from build123d import *

# Parameters (mm, degrees)
F0_W      = 232.5
F0_H      = 293
F1_DEPTH  = 200
F2_W      = 242.5
F2_H      = 5
F3_DEPTH  = 303
F5_DEPTH  = 25
F7_DEPTH  = 25
F9_DEPTH  = 210.001
F11_DEPTH = 210
F12_W     = 5
F12_H     = 82
F13_DEPTH = 232


with BuildPart() as f1:
    # F0 (on Front) → F1 (new body)
    with BuildSketch(Plane.XZ):
        Polygon((-92.2009944916, 239.5714490414), (-92.2009944916, 234.5714490414), (-92.2009944916, -63.4285509586), (150.2990055084, -63.4285509586), (150.2990055084, 239.5714490414), align=None)
        with Locations((29.0490055084, 88.0714490414)):
            Rectangle(F0_W, F0_H, mode=Mode.SUBTRACT)
    extrude(amount=F1_DEPTH)

    # F4 (on face) → F5 (cut)
    with BuildSketch(Plane.YZ.offset(150.2990055084)):
        with BuildLine():
            ThreePointArc((-42.5, 147.0714490414), (-44.6966991411, 152.3747499003), (-50, 154.5714490414))
            Line((-50, 154.5714490414), (-50, 147.0714490414))
            Line((-50, 147.0714490414), (-50, 139.5714490414))
            ThreePointArc((-50, 139.5714490414), (-44.6966991411, 141.7681481825), (-42.5, 147.0714490414))
        make_face()
        with BuildLine():
            ThreePointArc((-42.5, -24.9285509586), (-44.6966991411, -19.6252500997), (-50, -17.4285509586))
            Line((-50, -17.4285509586), (-50, -24.9285509586))
            Line((-50, -24.9285509586), (-50, -32.4285509586))
            ThreePointArc((-50, -32.4285509586), (-44.6966991411, -30.2318518175), (-42.5, -24.9285509586))
        make_face()
        with BuildLine():
            Line((-50, -24.9285509586), (-50, -17.4285509586))
            ThreePointArc((-50, -17.4285509586), (-57.5, -24.9285509586), (-50, -32.4285509586))
            Line((-50, -32.4285509586), (-50, -24.9285509586))
        make_face()
        with BuildLine():
            Line((-50, 147.0714490414), (-50, 154.5714490414))
            ThreePointArc((-50, 154.5714490414), (-57.5, 147.0714490414), (-50, 139.5714490414))
            Line((-50, 139.5714490414), (-50, 147.0714490414))
        make_face()
        with BuildLine():
            ThreePointArc((-142.5, 147.0714490414), (-144.6966991411, 152.3747499003), (-150, 154.5714490414))
            Line((-150, 154.5714490414), (-150, 147.0714490414))
            Line((-150, 147.0714490414), (-150, 139.5714490414))
            ThreePointArc((-150, 139.5714490414), (-144.6966991411, 141.7681481825), (-142.5, 147.0714490414))
        make_face()
        with BuildLine():
            ThreePointArc((-142.5, -24.9285509586), (-144.6966991411, -19.6252500997), (-150, -17.4285509586))
            Line((-150, -17.4285509586), (-150, -24.9285509586))
            Line((-150, -24.9285509586), (-150, -32.4285509586))
            ThreePointArc((-150, -32.4285509586), (-144.6966991411, -30.2318518175), (-142.5, -24.9285509586))
        make_face()
        with BuildLine():
            Line((-150, -24.9285509586), (-150, -17.4285509586))
            ThreePointArc((-150, -17.4285509586), (-157.5, -24.9285509586), (-150, -32.4285509586))
            Line((-150, -32.4285509586), (-150, -24.9285509586))
        make_face()
        with BuildLine():
            Line((-150, 147.0714490414), (-150, 154.5714490414))
            ThreePointArc((-150, 154.5714490414), (-157.5, 147.0714490414), (-150, 139.5714490414))
            Line((-150, 139.5714490414), (-150, 147.0714490414))
        make_face()
    extrude(amount=-F5_DEPTH, mode=Mode.SUBTRACT)

    # F6 (on face) → F7 (cut)
    with BuildSketch(Plane(origin=(0, 0, -63.4285509586), x_dir=(1, 0, 0), z_dir=(0, 0, -1))):
        with BuildLine():
            ThreePointArc((105.7990055084, 150), (113.2990055084, 142.5), (120.7990055084, 150))
            Line((120.7990055084, 150), (113.2990055084, 150))
            Line((113.2990055084, 150), (105.7990055084, 150))
        make_face()
        with BuildLine():
            Line((113.2990055084, 150), (120.7990055084, 150))
            ThreePointArc((120.7990055084, 150), (113.2990055084, 157.5), (105.7990055084, 150))
            Line((105.7990055084, 150), (113.2990055084, 150))
        make_face()
        with BuildLine():
            ThreePointArc((120.7990055084, 50), (113.2990055084, 57.5), (105.7990055084, 50))
            Line((105.7990055084, 50), (113.2990055084, 50))
            Line((113.2990055084, 50), (120.7990055084, 50))
        make_face()
        with BuildLine():
            Line((113.2990055084, 50), (105.7990055084, 50))
            ThreePointArc((105.7990055084, 50), (113.2990055084, 42.5), (120.7990055084, 50))
            Line((120.7990055084, 50), (113.2990055084, 50))
        make_face()
        with BuildLine():
            ThreePointArc((-19.2009944916, 50), (-21.3976936327, 55.3033008589), (-26.7009944916, 57.5))
            Line((-26.7009944916, 57.5), (-26.7009944916, 50))
            Line((-26.7009944916, 50), (-19.2009944916, 50))
        make_face()
        with BuildLine():
            Line((-26.7009944916, 50), (-26.7009944916, 57.5))
            ThreePointArc((-26.7009944916, 57.5), (-32.0042953505, 55.3033008589), (-34.2009944916, 50))
            Line((-34.2009944916, 50), (-26.7009944916, 50))
        make_face()
        with BuildLine():
            ThreePointArc((-26.7009944916, 142.5), (-21.3976936327, 144.6966991411), (-19.2009944916, 150))
            Line((-19.2009944916, 150), (-26.7009944916, 150))
            Line((-26.7009944916, 150), (-26.7009944916, 142.5))
        make_face()
        with BuildLine():
            Line((-26.7009944916, 150), (-19.2009944916, 150))
            ThreePointArc((-19.2009944916, 150), (-26.7009944916, 157.5), (-34.2009944916, 150))
            Line((-34.2009944916, 150), (-26.7009944916, 150))
        make_face()
        with BuildLine():
            Line((-26.7009944916, 142.5), (-26.7009944916, 150))
            Line((-26.7009944916, 150), (-34.2009944916, 150))
            ThreePointArc((-34.2009944916, 150), (-32.0042953505, 144.6966991411), (-26.7009944916, 142.5))
        make_face()
        with BuildLine():
            Line((-19.2009944916, 50), (-26.7009944916, 50))
            Line((-26.7009944916, 50), (-34.2009944916, 50))
            ThreePointArc((-34.2009944916, 50), (-26.7009944916, 42.5), (-19.2009944916, 50))
        make_face()
    extrude(amount=-F7_DEPTH, mode=Mode.SUBTRACT)



with BuildPart() as f3:
    # F2 (on face) → F3 (new body)
    with BuildSketch(Plane(origin=(0, 0, -63.4285509586), x_dir=(1, 0, 0), z_dir=(0, 0, -1))):
        with Locations((29.0490055084, 202.5)):
            Rectangle(F2_W, F2_H)
    extrude(amount=-F3_DEPTH)

    # F8 (on face) → F9 (cut, through all)
    with BuildSketch(Plane.XZ.offset(205)):
        with BuildLine():
            ThreePointArc((42.2990055084, 27.0714490414), (54.6733741792, 32.1970803706), (59.7990055084, 44.5714490414))
            ThreePointArc((59.7990055084, 44.5714490414), (29.9246368377, 56.9458177121), (42.2990055084, 27.0714490414))
        make_face()
    extrude(amount=-F9_DEPTH, mode=Mode.SUBTRACT)


with BuildPart() as f3b:
    # F2 (on face) → F3, piece 2 (new body)
    with BuildSketch(Plane(origin=(0, 0, -63.4285509586), x_dir=(1, 0, 0), z_dir=(0, 0, -1))):
        with Locations((29.0490055084, -2.5)):
            Rectangle(F2_W, F2_H)
    extrude(amount=-F3_DEPTH)


with BuildPart() as f1_1:
    add(f1.part)

    add(f3.part)  # F11 merges F3

    add(f3b.part)  # F11 merges F3b
    # F10 (on face) → F11 (join)
    with BuildSketch(Plane.XZ.offset(205)):
        Polygon((145.2990055084, -145.4285509586), (42.2990055084, -145.4285509586), (42.2990055084, -150.4285509586), (150.2990055084, -150.4285509586), (150.2990055084, -63.4285509586), (145.2990055084, -63.4285509586), align=None)
        Polygon((42.2990055084, -150.4285509586), (42.2990055084, -145.4285509586), (-87.2009944916, -145.4285509586), (-87.2009944916, -63.4285509586), (-92.2009944916, -63.4285509586), (-92.2009944916, -150.4285509586), align=None)
    extrude(amount=-F11_DEPTH)

    # F12 (on face) → F13 (join)
    with BuildSketch(Plane(origin=(145.2990055084, 0, 0), x_dir=(0, -1, 0), z_dir=(-1, 0, 0))):
        with Locations((-2.5, -104.4285509586)):
            Rectangle(F12_W, F12_H)
        with Locations((202.5, -104.4285509586)):
            Rectangle(F12_W, F12_H)
    extrude(amount=F13_DEPTH)


solid = f1_1.part
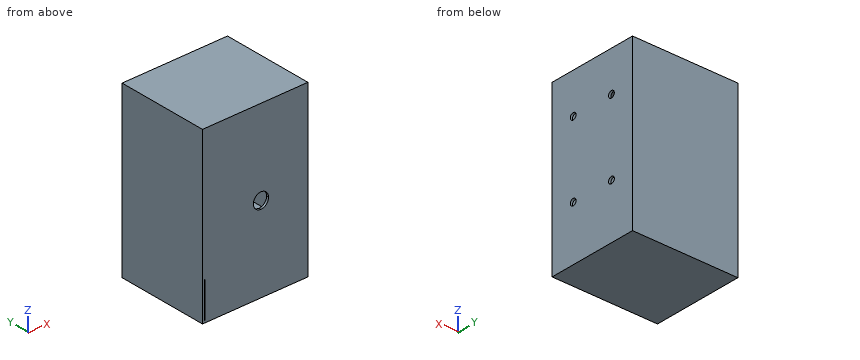
Could you check a few things on this model? Use its own coordinates, in mm. Give positions to 0.01 mm unless a question says otherwise; leave off trailing zeros. Write each loop counter-clockwise with the first axis right and the second up, starting at its lowest first coordinate (ties: lowest second). Pieces come first, ordered by that corner, then holes. Notation, with made-up numbers: (63.5, -20.5) -> (120.5, -20.5) arc R16 cw to (120.5, -10.5) -> close; hole circle Ø2 at (24, -2). An arc over 180 degrees is marked (long way). Answer as CSV lines item,"result". Start each with the question number.
(1) If we section it at C-C, the plane y = -92.5: Write out the boundary of the cut face in (x, z), and give its area (3 significant figures).
(2) I'm going to push a flat-ended pin straight in: pin 1 Ø12 at (y, z) = (-150, 147.07) entering from +X. Where does the tip first touch, or does it pass through?
(3) If we section it at D-D, the plane z = -116: Write out the boundary of the cut face in (x, y).
(4) If we section it at A-A, the plane z = 165: Write out the boundary of the cut face in (x, y), and give its area (4 significant figures).
(5) If we section it at B-B, the plane x = 130: Write out the boundary of the cut face in (y, z).
(6) Please list where these lines run through material, in increasing order: line 1 (Z direction, x = 124, y = -14); line 2 (Z direction, x = 149, y = -150); line 3 (Y direction, x = -1, z = 143.5).
Answer list:
1,outline,"(-92.2, -150.43) -> (150.3, -150.43) -> (150.3, 239.57) -> (-92.2, 239.57) -> close; hole (-87.2, -145.43) -> (145.3, -145.43) -> (145.3, -63.43) -> (-87.2, -63.43) -> close; hole (-87.2, -58.43) -> (145.3, -58.43) -> (145.3, 234.57) -> (-87.2, 234.57) -> close"
1,area,"7,390 mm^2"
2,pin 1,"x = -87.2"
3,outline,"(-92.2, -205) -> (-87.2, -205) -> (-87.2, 5) -> (-92.2, 5) -> close; (-86.7, -205) -> (150.3, -205) -> (150.3, 5) -> (-86.7, 5) -> (-86.7, 0) -> (145.3, 0) -> (145.3, -200) -> (-86.7, -200) -> close"
4,outline,"(-92.2, -205) -> (150.3, -205) -> (150.3, 5) -> (-92.2, 5) -> close; hole (-87.2, -200) -> (145.3, -200) -> (145.3, 0) -> (-87.2, 0) -> close"
4,area,"4,425 mm^2"
5,outline,"(-205, -150.43) -> (5, -150.43) -> (5, 239.57) -> (-205, 239.57) -> close; hole (-200, -145.43) -> (0, -145.43) -> (0, -63.43) -> (-200, -63.43) -> close; hole (-200, -58.43) -> (0, -58.43) -> (0, 234.57) -> (-200, 234.57) -> close"
6,line 1,"-150.43 to -145.43, -63.43 to -58.43, 234.57 to 239.57"
6,line 2,"-150.43 to -32.43, -17.43 to 139.57, 154.57 to 239.57"
6,line 3,"-205 to -200, 0 to 5"
